```python
from build123d import *

# Parameters (mm, degrees)
SKETCH1_R              = 113
SKETCH1_R_2            = 83
BOSS_EXTRUDE1_DEPTH    = 22.5
CHAMFER1_SIZE          = 3
M16X2_0_TAPPED_HOLE1_D = 14
CIRPATTERN1_COUNT      = 4


with BuildPart() as part:
    # Sketch1 → Boss-Extrude1 (new body, symmetric)
    with BuildSketch(Plane.XY):
        Circle(SKETCH1_R)
        Circle(SKETCH1_R_2, mode=Mode.SUBTRACT)
    extrude(amount=BOSS_EXTRUDE1_DEPTH, both=True)

    # Chamfer1
    chamfer1_edges = [part.edges().sort_by_distance(p)[0] for p in [
        (-113, 0, -22.5),
        (-113, 0, 22.5),
        (-83, 0, -22.5),
        (-83, 0, 22.5),
    ]]
    chamfer(chamfer1_edges, length=CHAMFER1_SIZE)

    # M16x2.0 Tapped Hole1 (through all)
    with Locations(Plane.XY.offset(22.5)):
        with Locations((-37.502976372, 90.540194186), (37.502976372, 90.540194186), (0, 98)):
            m16x2_0_tapped_hole1 = Hole(M16X2_0_TAPPED_HOLE1_D / 2)

    # CirPattern1: M16x2.0 Tapped Hole1 ×4 about axis
    cirpattern1_axis = Axis((0, 0, 0), (0, 0, 1))
    for i in range(1, CIRPATTERN1_COUNT):
        add(m16x2_0_tapped_hole1.rotate(cirpattern1_axis, i * 360 / CIRPATTERN1_COUNT), mode=Mode.SUBTRACT)


solid = part.part
```
Design review of the part built by this model. Coordinates are the model's own, in mm. Coordinates: 2 decimals unless noted, no trailing zeros. Loops run counter-clockwise (first coordinate to the right, second up) from the corner with the lowest first, then second, coordinate; pieces in that order, holes last.
Q1. The part is to be moulded in two halves that separate along X. For faces 1 (the face through (79.167, 24.931, -0.273)), 2 (the face through (60.75, 95.28, 0.27)), 3 (the face through (104.94, -0.91, -0.31)), 4 (the face through (-58, -65, 22.5)), say which applies: +X half, -X half, draft (parallel to the pull), parting line (faces both ways), or undercut.
Reported:
face 1: undercut
face 2: parting line
face 3: undercut
face 4: draft
Q2. For pin 1 (8.5 mm diameter, centred on x = -37.5, y = -90.54, fed in from -Z); pin 2 (1.5 mm diameter, centred on x = 6.5, z = -4, fed in from +Y); pin 3 (12 mm diameter, centred on x = 40, z = -16.5, fed in from +Y); pin 4 (3 mm diameter, centred on y = -79, z = 13, fed in from +X), all flat-tipped, find the tip position at first contact; note any pin that passes through.
Reported:
pin 1: passes through
pin 2: stops at y = 112.85
pin 3: stops at y = 107.76
pin 4: stops at x = 82.24
Q3. To check wall thickness, follow line 1 (Y direction, x = 1, z = 9.5); line 2 (X direction, y = 92, z = 0.5); line 3 (Y direction, x = -93, z = -16). State the ranges of each line that lie inside material, in increasing order.
Reported:
line 1: y = -113 to -104.93, -91.07 to -82.99, 82.99 to 91.07, 104.93 to 113
line 2: x = -65.61 to -44.35, -30.66 to -3.61, 3.61 to 30.66, 44.35 to 65.61
line 3: y = -64.19 to -44.06, -30.95 to -4.9, 4.9 to 30.95, 44.06 to 64.19
Q4. We need section A-A on y = 0. State the section outline as (x, z) points.
Reported:
outline: (-113, -19.5) - (-110, -22.5) - (-105, -22.5) - (-105, 22.5) - (-110, 22.5) - (-113, 19.5) - close; (-91, -22.5) - (-86, -22.5) - (-83, -19.5) - (-83, 19.5) - (-86, 22.5) - (-91, 22.5) - close; (83, -19.5) - (86, -22.5) - (91, -22.5) - (91, 22.5) - (86, 22.5) - (83, 19.5) - close; (105, -22.5) - (110, -22.5) - (113, -19.5) - (113, 19.5) - (110, 22.5) - (105, 22.5) - close
Q5. We need section C-C on z = 4. State how many separate pieces and enclosed holes the cut face has, and give its area (3 significant figures).
Reported:
separate pieces: 1
enclosed holes: 13
area: 16,600 mm2
